Read the model definition and answer for the solid it produces. Units are mm, in the model's axes. Face numbers are marked on the shaded views. A direction names the side the tool comes from. Round coordinates to 2 decimals unless told otherwise and drop trailing zeros. Loops run counter-clockwise (first coordinate to the right, second up) from the corner with the lowest first, then second, coordinate; pieces in that order, holes last. Notation, with made-up numbers: (-12.75, 78.5) -> (41.25, 78.5) arc R11 cw to (41.25, 95.5) -> close; hole circle Ø6 at (-6.5, -15). An arc over 180 degrees is marked (long way). Put each result on its own line as item: value.
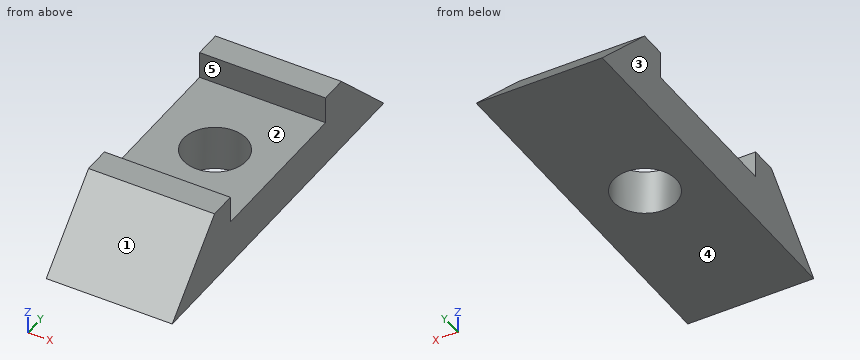
from build123d import *

# Parameters (mm, degrees)
F0_W     = 7
F0_H     = 20
F0_R     = 1.75
F1_DEPTH = 2.5
F2_W     = 7
F2_H     = 5.5
F3_DEPTH = 1.5
F4_SIZE  = 3.99999


# Not quite as in the source:
# - a fillet or chamfer is up to 0.001 mm smaller than in the source, because OpenCascade refuses the exact size


with BuildPart() as f1:
    # F0 (on Top) → F1 (new body)
    with BuildSketch(Plane.XY):
        Rectangle(F0_W, F0_H)
        Circle(F0_R, mode=Mode.SUBTRACT)
    extrude(amount=F1_DEPTH)

    # F2 (on face) → F3 (join)
    with BuildSketch(Plane.XY.offset(2.5)):
        with Locations((0, 7.25)):
            Rectangle(F2_W, F2_H)
        with Locations((0, -7.25)):
            Rectangle(F2_W, F2_H)
    extrude(amount=F3_DEPTH)

    # F4 (size 4 in the source; OpenCascade refuses exactly that, so slightly less here)
    f4_edges = [f1.edges().sort_by_distance(p)[0] for p in [
        (0, 10, 4),
        (0, -10, 4),
    ]]
    chamfer(f4_edges, length=F4_SIZE)


solid = f1.part
Item 1: Which of the six approach directions +Z, -Z, +X, -X, +Y, -Y give full straight-line access (tool end or side, diameter ignored) to the marked faces 4 and 5?
Derived:
face 4: -Z, +X, -X, +Y, -Y
face 5: +Z, +X, -X
Item 2: For a pull along Y with two mould halves and no side action, classify the marked faces 1, 2 and 3 as pulls with the +Y half, pulls with the -Y half, needs draft (parallel to the pull), parting line crosses it, or undercut.
Derived:
face 1: pulls with the -Y half
face 2: undercut
face 3: needs draft
Item 3: Find the intervals of material crossed by line 1 along Z through (x, y) = (1.25, 2.75); line 2 along Y through (x, z) = (0.75, 0.65); line 3 along Y through (x, z) = (0, 1.5), in increasing order.
Derived:
line 1: z = 0 to 2.5
line 2: y = -9.35 to -1.58, 1.58 to 9.35
line 3: y = -8.5 to -1.75, 1.75 to 8.5
Item 4: The part is cut by section C-C (y = 0). Determine the outline of the cut face in (x, z), then the cut area to 3 significant figures.
Derived:
outline: (-3.5, 0) -> (-1.75, 0) -> (-1.75, 2.5) -> (-3.5, 2.5) -> close; (1.75, 0) -> (3.5, 0) -> (3.5, 2.5) -> (1.75, 2.5) -> close
area: 8.75 mm^2
Item 5: Flat-ended cylindrical pins translate along their axes: pin 1 Ø1.5 at (x, z) = (-2.5, 0.5) entering from -Y; pin 2 Ø1.5 at (x, z) = (0, 1.5) entering from -Y; pin 3 Ø0.8 at (x, z) = (1.5, 3) entering from +Y. Find the tip coordinate at first contact, or state that the pin passes through.
Derived:
pin 1: stops at y = -10
pin 2: stops at y = -9.25
pin 3: stops at y = 7.4
Item 6: The part is cut by section D-D (z = 2.1). Determine the outline of the cut face in (x, y), then the cut area to 3 significant figures.
Derived:
outline: (-3.5, -7.9) -> (3.5, -7.9) -> (3.5, 7.9) -> (-3.5, 7.9) -> close; hole circle Ø3.5 at (0, 0)
area: 101 mm^2
Item 7: The part is cut by section A-A (z = 3.3). Determine the outline of the cut face in (x, y).
Derived:
outline: (-3.5, -6.7) -> (3.5, -6.7) -> (3.5, -4.5) -> (-3.5, -4.5) -> close; (-3.5, 4.5) -> (3.5, 4.5) -> (3.5, 6.7) -> (-3.5, 6.7) -> close
